Part model, mm, in its own coordinate system. Coordinates: 2 decimals unless noted, no trailing zeros. Order: outer loops, then holes, each group sorted by start corner. A loop starts at its lowest first (then second) coordinate and runs counter-clockwise, first axis right, second up.
1) Wall check: L1, parallel to X at y = 1, z = -19; L2, parallel to X at y = 3.5, z = -52.5; L3, parallel to Y at x = -3.5, z = -42. Give the ranges that are in metal, low to high.
2) Cut at C-C (x = 1.25). List the corners of the cut face in (y, z) (3 decimals).
3) Cut at A-A (z = -58). List the corners of the cut face in (x, y), and give its area (3 significant figures).
4) Cut at B-B (y = -3.75). List the corners of the cut face in (x, z) (1 decimal), and give its area (3 significant figures).
5) Cut at D-D (x = -4.5). List the corners of the cut face in (y, z) (3 decimals), and give its area (3 significant figures).
6) Pin check, flat tips, straight feed: pin 1 Ø5 at (x, y) = (-2, 2) entering from -Z (3 decimals); pin 2 Ø6 at (x, z) = (-2, 25) entering from +Y. Stop position of each tip, or through.
```python
from build123d import *

# Parameters (mm, degrees)
F0_W        = 11.557
F0_H        = 133.35
F0_W_2      = 6.604
F0_H_2      = 127
F0_W_3      = 3.175
F1_DEPTH    = 5.08
F2_T1_DEPTH = 5.08
F3_DEPTH    = 4.7625
F5_DEPTH    = 133.351


# Not quite as in the source:
# - a fillet or chamfer that OpenCascade refuses, or shapes differently, is made with other operations: its cross-section is extruded or revolved along the edge and cut away or added


with BuildPart() as f1:
    # F0 (on Front) → F1 (new body)
    with BuildSketch(Plane.XZ):
        Rectangle(F0_W, F0_H)
        Rectangle(F0_W_2, F0_H_2, mode=Mode.SUBTRACT)
        with Locations((-7.366, 0)):
            Rectangle(F0_W_3, F0_H)
        with Locations((7.366, 0)):
            Rectangle(F0_W_3, F0_H)
    extrude(amount=F1_DEPTH)

    # F2: fillet of radius 3.429 on 4 edges, made by hand

    # F2_s2 → F2_t1 (join)
    with BuildSketch(Plane.XZ):
        with BuildLine():
            ThreePointArc((-0.127, 63.5), (2.2976691527, 62.4956691527), (3.302, 60.071))
            Line((3.302, 60.071), (3.302, 63.5))
            Line((3.302, 63.5), (-0.127, 63.5))
        make_face()
        with BuildLine():
            ThreePointArc((-3.302, 60.071), (-2.2976691527, 62.4956691527), (0.127, 63.5))
            Line((0.127, 63.5), (-3.302, 63.5))
            Line((-3.302, 63.5), (-3.302, 60.071))
        make_face()
        with BuildLine():
            ThreePointArc((0.127, -63.5), (-2.2976691527, -62.4956691527), (-3.302, -60.071))
            Line((-3.302, -60.071), (-3.302, -63.5))
            Line((-3.302, -63.5), (0.127, -63.5))
        make_face()
        with BuildLine():
            ThreePointArc((-0.127, -63.5), (2.2976691527, -62.4956691527), (3.302, -60.071))
            Line((3.302, -60.071), (3.302, -63.5))
            Line((3.302, -63.5), (-0.127, -63.5))
        make_face()
    extrude(amount=F2_T1_DEPTH)

    # F0 (on Front) → F3 (join)
    with BuildSketch(Plane.XZ):
        with Locations((7.366, 0)):
            Rectangle(F0_W_3, F0_H)
        with Locations((-7.366, 0)):
            Rectangle(F0_W_3, F0_H)
    extrude(amount=-F3_DEPTH)

    # F4 (on face) → F5 (cut, through all)
    with BuildSketch(Plane.XY.offset(66.675)):
        with BuildLine():
            ThreePointArc((-8.9535, -0.06985), (-8.3428425838, 0.1830925838), (-8.0899, 0.79375))
            ThreePointArc((-8.0899, 0.79375), (-8.3428425838, 1.4044074162), (-8.9535, 1.65735))
            Line((-8.9535, 1.65735), (-8.9535, -0.06985))
        make_face()
        with BuildLine():
            ThreePointArc((-8.0899, -1.11125), (-8.3428425838, -0.5005925838), (-8.9535, -0.24765))
            Line((-8.9535, -0.24765), (-8.9535, -1.97485))
            ThreePointArc((-8.9535, -1.97485), (-8.3428425838, -1.7219074162), (-8.0899, -1.11125))
        make_face()
        with BuildLine():
            ThreePointArc((8.9535, -0.24765), (8.0899, -1.11125), (8.9535, -1.97485))
            Line((8.9535, -1.97485), (8.9535, -0.24765))
        make_face()
        with BuildLine():
            Line((8.9535, -0.06985), (8.9535, 1.65735))
            ThreePointArc((8.9535, 1.65735), (8.0899, 0.79375), (8.9535, -0.06985))
        make_face()
    extrude(amount=-F5_DEPTH, mode=Mode.SUBTRACT)


solid = f1.part
```
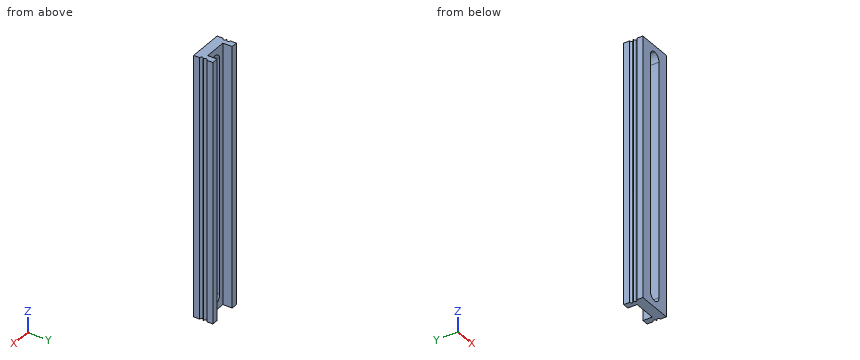
Geometry check:
1. L1: x = -8.11 to -5.78, 5.78 to 8.11
1. L2: x = -8.95 to -5.78, 5.78 to 8.95
1. L3: y = -5.08 to 0
2. outline: (-5.08, -66.675) - (0, -66.675) - (0, -63.211) - (-5.08, -63.211) - close; (-5.08, 63.211) - (0, 63.211) - (0, 66.675) - (-5.08, 66.675) - close
3. outline: (-8.95, -5.08) - (-3.3, -5.08) - (-3.3, 0) - (-5.78, 0) - (-5.78, 4.76) - (-8.95, 4.76) - (-8.95, 1.66) arc R0.86 cw to (-8.95, -0.07) - (-8.95, -0.25) arc R0.86 cw to (-8.95, -1.97) - close; (3.3, -5.08) - (8.95, -5.08) - (8.95, -1.97) arc R0.86 cw to (8.95, -0.25) - (8.95, -0.07) arc R0.86 cw to (8.95, 1.66) - (8.95, 4.76) - (5.78, 4.76) - (5.78, 0) - (3.3, 0) - close
3. area: 83.0 mm2
4. outline: (-9, -66.7) - (9, -66.7) - (9, 66.7) - (-9, 66.7) - close; hole (-3.3, -60.1) arc R3.4 ccw to (0, -63.5) arc R3.4 ccw to (3.3, -60.1) - (3.3, 60.1) arc R3.4 ccw to (0, 63.5) arc R3.4 ccw to (-3.3, 60.1) - close
4. area: 1,560 mm2
5. outline: (-5.08, -66.675) - (0, -66.675) - (0, 66.675) - (-5.08, 66.675) - close
5. area: 677 mm2
6. pin 1: stops at z = -66.675
6. pin 2: stops at y = 0
